Check sheet for the modelled part. Datum: model origin and axes. Units: mm. Give positions to 0.01 mm unless a question says otherwise; leave off trailing zeros. Order: outer loops, then holes, each group sorted by start corner. A loop starts at its lowest first (then second) coordinate and runs counter-clockwise, first axis right, second up. Notation, with made-up numbers: (12, 70) -> (16, 70) arc R16 ccw to (16, 86) -> close; hole circle Ø9 at (-39.5, 76.5). An arc over 180 degrees is marked (long way). Answer in a Markdown table with one row per item. Add a question column.
(1) Cross-section at B-B (x = 118.5). Record the cut outline in (y, z).
(2) Thickness scan on L1, parallel to Z at x = 218.5, y = 58.1; L2, parallel to X at y = 58.6, z = -80. Record the ranges inside material, lowest first. Write a range as [from, to].
(3) Go/stop test with flat-tipped pins: pin 1 (1.5 mm diameter, centred on y = 58.5, z = 2, fed in from +X); pin 2 (1 mm diameter, centred on y = 58, z = -27, fed in from -X); pin 3 (0.9 mm diameter, centred on y = 58, z = -95, fed in from -X). Record where each tip stops, or that it passes through.
(4) Cross-section at A-A (z = -71). Record the cut outline in (x, y).
Autodesk Inventor part; units mm, degrees
ref_plane "Work Plane1" through (127, 57.2, 0) normal (0, 1, 0) x (1, 0, 0)
ref_plane "YZ Plane" through (0, 0, 0) normal (1, 0, 0) x (0, 1, 0)
ref_plane "XZ Plane" through (0, 0, 0) normal (0, 1, 0) x (-1, 0, 0)
ref_plane "Work Plane1" through (127, 57.2, 0) normal (0, 1, 0) x (1, 0, 0)
sketch "Sketch3" plane through (127, 57.2, 0) normal (0, 1, 0) x (1, 0, 0)
  line L0 (0, 0) -> (85, 0) construction
  line L1 (0, 0) -> (0, -3) construction
  line L2 (85, -3) -> (0, -3) construction
  line L3 (85, 0) -> (85, -3) construction
  line L4 (-102, 0) -> (-17, 0) construction
  line L5 (-102, 0) -> (-102, -3) construction
  line L6 (-17, -3) -> (-102, -3) construction
  line L7 (-17, 0) -> (-17, -3) construction
  line L8 (122, 10) -> (125, 10) construction
  line L9 (122, 10) -> (122, 0) construction
  line L10 (125, 0) -> (122, 0) construction
  line L11 (125, 10) -> (125, 0) construction
  line L12 (122, 40) -> (125, 40) construction
  line L13 (125, 54) -> (125, 40) construction
  line L14 (122, 54) -> (125, 54) construction
  line L15 (122, 54) -> (122, 40) construction
  line L16 (122, 84) -> (125, 84) construction
  line L17 (125, 94) -> (125, 84) construction
  line L18 (122, 94) -> (125, 94) construction
  line L19 (122, 94) -> (122, 84) construction
  line L20 (122, 0) -> (-139, 0)
  line L21 (-139, 0) -> (-139, 94)
  line L22 (-139, 94) -> (122, 94)
  line L23 (122, 94) -> (122, 0)
  line L24 (-102, 0) -> (-142, 0)
  line L25 (-17, -3) -> (-102, -3)
  line L26 (-102, -3) -> (-102, 0)
  line L27 (-102, 0) -> (-17, 0)
  line L28 (-17, 0) -> (-17, -3)
  line L29 (85, -3) -> (0, -3)
  line L30 (0, -3) -> (0, 0)
  line L31 (0, 0) -> (85, 0)
  line L32 (85, 0) -> (85, -3)
  line L33 (122, 10) -> (125, 10)
  line L34 (122, 0) -> (125, 0)
  line L35 (125, 0) -> (125, 10)
  line L36 (125, 10) -> (122, 10)
  line L37 (122, 10) -> (122, 0)
  line L38 (125, 54) -> (125, 40)
  line L39 (122, 40) -> (125, 40)
  line L40 (125, 40) -> (125, 54)
  line L41 (125, 54) -> (122, 54)
  line L42 (122, 54) -> (122, 40)
  line L43 (122, 94) -> (125, 94)
  line L44 (125, 94) -> (125, 84)
  line L45 (125, 84) -> (122, 84)
  line L46 (122, 84) -> (122, 94)
  line L47 (-139, 47) -> (122, 47) construction
  line L48 (-8.5, 94) -> (-8.5, 0) construction
  line L49 (-139, 10) -> (-142, 10) construction
  line L50 (-139, 10) -> (-139, 0) construction
  line L51 (-142, 0) -> (-139, 0) construction
  line L52 (-142, 10) -> (-142, 0) construction
  line L53 (-139, 40) -> (-142, 40) construction
  line L54 (-142, 54) -> (-142, 40) construction
  line L55 (-139, 54) -> (-142, 54) construction
  line L56 (-139, 54) -> (-139, 40) construction
  line L57 (-139, 84) -> (-142, 84) construction
  line L58 (-142, 94) -> (-142, 84) construction
  line L59 (-139, 94) -> (-142, 94) construction
  line L60 (-139, 94) -> (-139, 84) construction
  line L61 (-139, 94) -> (-139, 0)
  line L62 (-139, 10) -> (-142, 10)
  line L63 (-139, 0) -> (-142, 0)
  line L64 (-142, 0) -> (-142, 10)
  line L65 (-142, 10) -> (-139, 10)
  line L66 (-139, 10) -> (-139, 0)
  line L67 (-142, 54) -> (-142, 40)
  line L68 (-139, 40) -> (-142, 40)
  line L69 (-142, 40) -> (-142, 54)
  line L70 (-142, 54) -> (-139, 54)
  line L71 (-139, 54) -> (-139, 40)
  line L72 (-139, 94) -> (-142, 94)
  line L73 (-142, 94) -> (-142, 84)
  line L74 (-142, 84) -> (-139, 84)
  line L75 (-139, 84) -> (-139, 94)
  line L76 (0, 94) -> (85, 94) construction
  line L77 (0, 94) -> (0, 97) construction
  line L78 (85, 97) -> (0, 97) construction
  line L79 (85, 94) -> (85, 97) construction
  line L80 (-102, 94) -> (-17, 94) construction
  line L81 (-102, 94) -> (-102, 97) construction
  line L82 (-17, 97) -> (-102, 97) construction
  line L83 (-17, 94) -> (-17, 97) construction
  line L84 (-17, 97) -> (-102, 97)
  line L85 (-102, 97) -> (-102, 94)
  line L86 (-102, 94) -> (-17, 94)
  line L87 (-17, 94) -> (-17, 97)
  line L88 (85, 97) -> (0, 97)
  line L89 (0, 97) -> (0, 94)
  line L90 (0, 94) -> (85, 94)
  line L91 (85, 94) -> (85, 97)
  point P0 (-127, 0)
  dimension "d55" = 261
  dimension "d56" = 94
extrude "Extrusion4" add sketch "Sketch3" along normal blind 3
properties part number "case_roof"
Answer below:
| question | item | result |
|---|---|---|
| 1 | outline | (57.2, -94) -> (60.2, -94) -> (60.2, 0) -> (57.2, 0) -> close |
| 2 | L1 | z = [-94, 0] |
| 2 | L2 | x = [-12, 249] |
| 3 | pin 1 | stops at x = 212 |
| 3 | pin 2 | stops at x = -12 |
| 3 | pin 3 | stops at x = 25 |
| 4 | outline | (-12, 57.2) -> (249, 57.2) -> (249, 60.2) -> (-12, 60.2) -> close |
